The listing builds one solid part. Answer for the finished solid, in the listing's coordinates (mm). A direction names the side the tool comes from. Give positions to 0.01 mm unless a question says otherwise; leave off trailing zeros. Loops run counter-clockwise (first coordinate to the right, second up) from the corner with the lowest first, then second, coordinate; pieces in that order, holes last. Notation, with made-up numbers: (60, -35) - (94, -35) arc R33 ccw to (94, -5) - close; hole circle Ø1 at (-30.75, 52.25). An arc over 180 degrees is marked (long way). Write each question's results on one line, items separated by ' | '.
from build123d import *

# Parameters (mm, degrees)
CYLINDER002_R     = 1.65
CYLINDER002_DEPTH = 10
BOX005_W          = 7
BOX005_H          = 5
BOX005_DEPTH      = 12
BOX006_W          = 14
BOX006_H          = 3
BOX006_DEPTH      = 12
BOX007_W          = 2
BOX007_H          = 5
BOX007_DEPTH      = 12
BOX008_W          = 14
BOX008_H          = 3
BOX008_DEPTH      = 12
BOX009_W          = 2
BOX009_H          = 5
BOX009_DEPTH      = 12
BOX010_W          = 7
BOX010_H          = 2
BOX010_DEPTH      = 7.8
CHAMFER005_SIZE   = 1


with BuildPart() as cylinder002:
    # Cylinder002 → Cylinder002 (new body)
    with BuildSketch(Plane(origin=(0, 0, 6), x_dir=(1, 0, 0), z_dir=(0, 1, 0))):
        Circle(CYLINDER002_R)
    extrude(amount=CYLINDER002_DEPTH)


with BuildPart() as cube005:
    # Box005 → Box005 (new body)
    with BuildSketch(Plane(origin=(-3.5, 0, 0), x_dir=(1, 0, 0), z_dir=(0, 0, 1))):
        with Locations((3.5, 2.5)):
            Rectangle(BOX005_W, BOX005_H)
    extrude(amount=BOX005_DEPTH)


with BuildPart() as cube006:
    # Box006 → Box006 (new body)
    with BuildSketch(Plane(origin=(3.5, 0, 0), x_dir=(1, 0, 0), z_dir=(0, 0, 1))):
        with Locations((7, 1.5)):
            Rectangle(BOX006_W, BOX006_H)
    extrude(amount=BOX006_DEPTH)


with BuildPart() as cube007:
    # Box007 → Box007 (new body)
    with BuildSketch(Plane(origin=(17.5, 0, 0), x_dir=(1, 0, 0), z_dir=(0, 0, 1))):
        with Locations((1, 2.5)):
            Rectangle(BOX007_W, BOX007_H)
    extrude(amount=BOX007_DEPTH)


with BuildPart() as cube008:
    # Box008 → Box008 (new body)
    with BuildSketch(Plane(origin=(-17.5, 0, 0), x_dir=(1, 0, 0), z_dir=(0, 0, 1))):
        with Locations((7, 1.5)):
            Rectangle(BOX008_W, BOX008_H)
    extrude(amount=BOX008_DEPTH)


with BuildPart() as cube009:
    # Box009 → Box009 (new body)
    with BuildSketch(Plane(origin=(-19.5, 0, 0), x_dir=(1, 0, 0), z_dir=(0, 0, 1))):
        with Locations((1, 2.5)):
            Rectangle(BOX009_W, BOX009_H)
    extrude(amount=BOX009_DEPTH)


with BuildPart() as chamfer005:
    # Box010 → Box010 (new body)
    with BuildSketch(Plane(origin=(-3.5, 4, 2.1), x_dir=(1, 0, 0), z_dir=(0, 0, 1))):
        with Locations((3.5, 1)):
            Rectangle(BOX010_W, BOX010_H)
    extrude(amount=BOX010_DEPTH)

    # Fusion003: union Cube005, Cube006, Cube007, Cube008, Cube009
    add(cube005.part)
    add(cube006.part)
    add(cube007.part)
    add(cube008.part)
    add(cube009.part)

    # Cut003: cut Cylinder002
    add(cylinder002.part, mode=Mode.SUBTRACT)

    # Chamfer005
    chamfer005_edges = [chamfer005.edges().sort_by_distance(p)[0] for p in [
        (-19.5, 0, 6),
        (19.5, 0, 6),
    ]]
    chamfer(chamfer005_edges, length=CHAMFER005_SIZE)


solid = chamfer005.part
Item 1: Flat-ended cylindrical pins translate along their axes: P1, Ø0.5, axis at x = -1.5, y = 5.5, coming from the -Z side; P2, Ø0.6, axis at x = 18.5, z = 6, coming from the +Y side; P3, Ø0.5, axis at x = 0.5, y = 5.5, coming from the +Z side. Find the tip coordinate at first contact, or state that the pin passes through.
Values found:
P1: stops at z = 2.1 | P2: stops at y = 5 | P3: stops at z = 9.9
Item 2: A cutting plane is placed at D-D, the plane y = 0.65. Determine the outline of the cut face in (x, z), plus the area to 3 significant figures.
Values found:
outline: (-19.15, 0) - (19.15, 0) - (19.15, 12) - (-19.15, 12) - close; hole circle Ø3.3 at (0, 6) | area: 451 mm²
Item 3: Find the intervals of material crossed by line 1 along X through (y, z) = (3.65, 3.5); line 2 along X through (y, z) = (1.6, 6); line 3 along Z through (x, y) = (0, 2.65), in increasing order. Write a range as [from, to].
Values found:
line 1: x = [-19.5, -17.5], [-3.5, 3.5], [17.5, 19.5] | line 2: x = [-19.5, -1.65], [1.65, 19.5] | line 3: z = [0, 4.35], [7.65, 12]
Item 4: A cutting plane is placed at C-C, the plane z = 6. Determine the outline of the cut face in (x, y).
Values found:
outline: (-19.5, 1) - (-18.5, 0) - (-1.65, 0) - (-1.65, 6) - (-3.5, 6) - (-3.5, 3) - (-17.5, 3) - (-17.5, 5) - (-19.5, 5) - close; (1.65, 0) - (18.5, 0) - (19.5, 1) - (19.5, 5) - (17.5, 5) - (17.5, 3) - (3.5, 3) - (3.5, 6) - (1.65, 6) - close
Item 5: For a pull along X with two mould halves and no side action, classify faces 1 (the face through (-19.5, 3, 6)), 2 (the face through (-19, 5, 6)), 3 (the face through (-11, 3, 6)), 4 (the face through (19, 0.5, 5.9)) as released by +X, released by -X, zero draft, split by the parting line, or undercut.
Values found:
face 1: released by -X | face 2: zero draft | face 3: undercut | face 4: released by +X
Item 6: For faces 5 (the face through (10, 3, 6)), 6 (the face through (0, 5, 1)), 7 (the face through (18, 5, 6)), 8 (the face through (0, 5.5, 9.9)), determine the directions among +Z, -Z, +X, -X, +Y, -Y from which every point of the face is accessible in a straight line to the end or side of a thin tool.
Values found:
face 5: +Z, -Z, +Y | face 6: -Z, +X, -X, +Y | face 7: +Z, -Z, +X, +Y | face 8: +Z, +X, -X, +Y
Item 7: A cutting plane is placed at A-A, the plane y = 3.35. Determine the outline of the cut face in (x, z).
Values found:
outline: (-19.5, 0) - (-17.5, 0) - (-17.5, 12) - (-19.5, 12) - close; (-3.5, 0) - (3.5, 0) - (3.5, 12) - (-3.5, 12) - close; (17.5, 0) - (19.5, 0) - (19.5, 12) - (17.5, 12) - close; hole circle Ø3.3 at (0, 6)
Item 8: A cutting plane is placed at B-B, the plane x = 0. Determine the outline of the cut face in (y, z).
Values found:
outline: (0, 0) - (5, 0) - (5, 2.1) - (6, 2.1) - (6, 4.35) - (0, 4.35) - close; (0, 7.65) - (6, 7.65) - (6, 9.9) - (5, 9.9) - (5, 12) - (0, 12) - close
